The listing builds one solid part. Answer for the finished solid, in the listing's coordinates (mm). Give positions to 0.01 mm unless a question says otherwise; leave off trailing zeros.
```python
from build123d import *

# Parameters (mm, degrees)
SKETCH4_W              = 100
SKETCH4_H              = 50
BODY_DEPTH             = 500
CUT_PROFILE_DEPTH      = 257.173769149
CUT_PROFILE_DEPTH_BACK = 257.173769149
SKETCH6_OUTSIDE_W      = 204.47
SKETCH6_OUTSIDE_H      = 154.47
SKETCH6_OUTSIDE_R      = 4.25
SKETCH6_OUTSIDE_R_2    = 2.5


with BuildPart() as part:
    # Sketch4 → Body (new body)
    with BuildSketch(Plane.XY.offset(250)):
        Rectangle(SKETCH4_W, SKETCH4_H)
    extrude(amount=-BODY_DEPTH)

    # Sketch6 outside → Cut-Profile (cut, two sides: drawn at the far end of the back side and taken through both)
    # profile 1 of 8: a face of its own
    with BuildSketch(Plane.XY.offset(-CUT_PROFILE_DEPTH_BACK)):
        Rectangle(SKETCH6_OUTSIDE_W, SKETCH6_OUTSIDE_H)
        with BuildLine():
            Line((-31.4, -19.7), (-35.8, -19.7))
            ThreePointArc((-35.8, -19.7), (-37.371513222, -18.648341109), (-36.998678382, -16.794524933))
            Line((-36.998678382, -16.794524933), (-31.125524653, -10.954485098))
            ThreePointArc((-31.125524653, -10.954485098), (-29.506885614, -9.877902288), (-27.6, -9.5))
            Line((-27.6, -9.5), (-22.4, -9.5))
            ThreePointArc((-22.4, -9.5), (-20.493114386, -9.877902288), (-18.874475347, -10.954485098))
            Line((-18.874475347, -10.954485098), (-13.001321618, -16.794524933))
            ThreePointArc((-13.001321618, -16.794524933), (-12.628486778, -18.648341109), (-14.2, -19.7))
            Line((-14.2, -19.7), (-18.6, -19.7))
            ThreePointArc((-18.6, -19.7), (-19.589949494, -20.110050506), (-20, -21.1))
            Line((-20, -21.1), (-20, -23.2))
            ThreePointArc((-20, -23.2), (-19.472792206, -24.472792206), (-18.2, -25))
            Line((-18.2, -25), (18.2, -25))
            ThreePointArc((18.2, -25), (19.472792206, -24.472792206), (20, -23.2))
            Line((20, -23.2), (20, -21.1))
            ThreePointArc((20, -21.1), (19.589949494, -20.110050506), (18.6, -19.7))
            Line((18.6, -19.7), (14.2, -19.7))
            ThreePointArc((14.2, -19.7), (12.628486778, -18.648341109), (13.001321618, -16.794524933))
            Line((13.001321618, -16.794524933), (18.874475347, -10.954485098))
            ThreePointArc((18.874475347, -10.954485098), (20.493114386, -9.877902288), (22.4, -9.5))
            Line((22.4, -9.5), (27.6, -9.5))
            ThreePointArc((27.6, -9.5), (29.506885614, -9.877902288), (31.125524653, -10.954485098))
            Line((31.125524653, -10.954485098), (36.998678382, -16.794524933))
            ThreePointArc((36.998678382, -16.794524933), (37.371513222, -18.648341109), (35.8, -19.7))
            Line((35.8, -19.7), (31.4, -19.7))
            ThreePointArc((31.4, -19.7), (30.410050506, -20.110050506), (30, -21.1))
            Line((30, -21.1), (30, -23.2))
            ThreePointArc((30, -23.2), (30.527207794, -24.472792206), (31.8, -25))
            Line((31.8, -25), (45, -25))
            ThreePointArc((45, -25), (48.535533906, -23.535533906), (50, -20))
            Line((50, -20), (50, -6.8))
            ThreePointArc((50, -6.8), (49.472792206, -5.527207794), (48.2, -5))
            Line((48.2, -5), (46.1, -5))
            ThreePointArc((46.1, -5), (45.110050506, -5.410050506), (44.7, -6.4))
            Line((44.7, -6.4), (44.7, -10.8))
            ThreePointArc((44.7, -10.8), (43.648341109, -12.371513222), (41.794524933, -11.998678382))
            Line((41.794524933, -11.998678382), (35.954485098, -6.125524653))
            ThreePointArc((35.954485098, -6.125524653), (34.877902288, -4.506885614), (34.5, -2.6))
            Line((34.5, -2.6), (34.5, 2.6))
            ThreePointArc((34.5, 2.6), (34.877902288, 4.506885614), (35.954485098, 6.125524653))
            Line((35.954485098, 6.125524653), (41.794524933, 11.998678382))
            ThreePointArc((41.794524933, 11.998678382), (43.648341109, 12.371513222), (44.7, 10.8))
            Line((44.7, 10.8), (44.7, 6.4))
            ThreePointArc((44.7, 6.4), (45.110050506, 5.410050506), (46.1, 5))
            Line((46.1, 5), (48.2, 5))
            ThreePointArc((48.2, 5), (49.472792206, 5.527207794), (50, 6.8))
            Line((50, 6.8), (50, 20))
            ThreePointArc((50, 20), (48.535533906, 23.535533906), (45, 25))
            Line((45, 25), (31.8, 25))
            ThreePointArc((31.8, 25), (30.527207794, 24.472792206), (30, 23.2))
            Line((30, 23.2), (30, 21.1))
            ThreePointArc((30, 21.1), (30.410050506, 20.110050506), (31.4, 19.7))
            Line((31.4, 19.7), (35.8, 19.7))
            ThreePointArc((35.8, 19.7), (37.371513222, 18.648341109), (36.998678382, 16.794524933))
            Line((36.998678382, 16.794524933), (31.125524653, 10.954485098))
            ThreePointArc((31.125524653, 10.954485098), (29.506885614, 9.877902288), (27.6, 9.5))
            Line((27.6, 9.5), (22.4, 9.5))
            ThreePointArc((22.4, 9.5), (20.493114386, 9.877902288), (18.874475347, 10.954485098))
            Line((18.874475347, 10.954485098), (13.001321618, 16.794524933))
            ThreePointArc((13.001321618, 16.794524933), (12.628486778, 18.648341109), (14.2, 19.7))
            Line((14.2, 19.7), (18.6, 19.7))
            ThreePointArc((18.6, 19.7), (19.589949494, 20.110050506), (20, 21.1))
            Line((20, 21.1), (20, 23.2))
            ThreePointArc((20, 23.2), (19.472792206, 24.472792206), (18.2, 25))
            Line((18.2, 25), (-18.2, 25))
            ThreePointArc((-18.2, 25), (-19.472792206, 24.472792206), (-20, 23.2))
            Line((-20, 23.2), (-20, 21.1))
            ThreePointArc((-20, 21.1), (-19.589949494, 20.110050506), (-18.6, 19.7))
            Line((-18.6, 19.7), (-14.2, 19.7))
            ThreePointArc((-14.2, 19.7), (-12.628486778, 18.648341109), (-13.001321618, 16.794524933))
            Line((-13.001321618, 16.794524933), (-18.874475347, 10.954485098))
            ThreePointArc((-18.874475347, 10.954485098), (-20.493114386, 9.877902288), (-22.4, 9.5))
            Line((-22.4, 9.5), (-27.6, 9.5))
            ThreePointArc((-27.6, 9.5), (-29.506885614, 9.877902288), (-31.125524653, 10.954485098))
            Line((-31.125524653, 10.954485098), (-36.998678382, 16.794524933))
            ThreePointArc((-36.998678382, 16.794524933), (-37.371513222, 18.648341109), (-35.8, 19.7))
            Line((-35.8, 19.7), (-31.4, 19.7))
            ThreePointArc((-31.4, 19.7), (-30.410050506, 20.110050506), (-30, 21.1))
            Line((-30, 21.1), (-30, 23.2))
            ThreePointArc((-30, 23.2), (-30.527207794, 24.472792206), (-31.8, 25))
            Line((-31.8, 25), (-45, 25))
            ThreePointArc((-45, 25), (-48.535533906, 23.535533906), (-50, 20))
            Line((-50, 20), (-50, 6.8))
            ThreePointArc((-50, 6.8), (-49.472792206, 5.527207794), (-48.2, 5))
            Line((-48.2, 5), (-46.1, 5))
            ThreePointArc((-46.1, 5), (-45.110050506, 5.410050506), (-44.7, 6.4))
            Line((-44.7, 6.4), (-44.7, 10.8))
            ThreePointArc((-44.7, 10.8), (-43.648341109, 12.371513222), (-41.794524933, 11.998678382))
            Line((-41.794524933, 11.998678382), (-35.954485098, 6.125524653))
            ThreePointArc((-35.954485098, 6.125524653), (-34.877902288, 4.506885614), (-34.5, 2.6))
            Line((-34.5, 2.6), (-34.5, -2.6))
            ThreePointArc((-34.5, -2.6), (-34.877902288, -4.506885614), (-35.954485098, -6.125524653))
            Line((-35.954485098, -6.125524653), (-41.794524933, -11.998678382))
            ThreePointArc((-41.794524933, -11.998678382), (-43.648341109, -12.371513222), (-44.7, -10.8))
            Line((-44.7, -10.8), (-44.7, -6.4))
            ThreePointArc((-44.7, -6.4), (-45.110050506, -5.410050506), (-46.1, -5))
            Line((-46.1, -5), (-48.2, -5))
            ThreePointArc((-48.2, -5), (-49.472792206, -5.527207794), (-50, -6.8))
            Line((-50, -6.8), (-50, -20))
            ThreePointArc((-50, -20), (-48.535533906, -23.535533906), (-45, -25))
            Line((-45, -25), (-31.8, -25))
            ThreePointArc((-31.8, -25), (-30.527207794, -24.472792206), (-30, -23.2))
            Line((-30, -23.2), (-30, -21.1))
            ThreePointArc((-30, -21.1), (-30.410050506, -20.110050506), (-31.4, -19.7))
        make_face(mode=Mode.SUBTRACT)
    # profile 2 of 8: a face of its own
    with BuildSketch(Plane.XY.offset(-CUT_PROFILE_DEPTH_BACK)):
        with Locations((25, 0)):
            Circle(SKETCH6_OUTSIDE_R)
    # profile 3 of 8: a face of its own
    with BuildSketch(Plane.XY.offset(-CUT_PROFILE_DEPTH_BACK)):
        with Locations((45, -20)):
            Circle(SKETCH6_OUTSIDE_R_2)
    # profile 4 of 8: a face of its own
    with BuildSketch(Plane.XY.offset(-CUT_PROFILE_DEPTH_BACK)):
        with Locations((45, 20)):
            Circle(SKETCH6_OUTSIDE_R_2)
    # profile 5 of 8: a face of its own
    with BuildSketch(Plane.XY.offset(-CUT_PROFILE_DEPTH_BACK)):
        with Locations((-45, -20)):
            Circle(SKETCH6_OUTSIDE_R_2)
    # profile 6 of 8: a face of its own
    with BuildSketch(Plane.XY.offset(-CUT_PROFILE_DEPTH_BACK)):
        with Locations((-45, 20)):
            Circle(SKETCH6_OUTSIDE_R_2)
    # profile 7 of 8: a face of its own
    with BuildSketch(Plane.XY.offset(-CUT_PROFILE_DEPTH_BACK)):
        with Locations((-25, 0)):
            Circle(SKETCH6_OUTSIDE_R)
    # profile 8 of 8: a face of its own
    with BuildSketch(Plane.XY.offset(-CUT_PROFILE_DEPTH_BACK)):
        with BuildLine():
            Line((14.914213562, 5.685786438), (1.555634919, 19.044365081))
            ThreePointArc((1.555634919, 19.044365081), (0, 19.688730163), (-1.555634919, 19.044365081))
            Line((-1.555634919, 19.044365081), (-14.914213562, 5.685786438))
            ThreePointArc((-14.914213562, 5.685786438), (-15.347759065, 5.03693974), (-15.5, 4.271572875))
            Line((-15.5, 4.271572875), (-15.5, -4.271572875))
            ThreePointArc((-15.5, -4.271572875), (-15.347759065, -5.03693974), (-14.914213562, -5.685786438))
            Line((-14.914213562, -5.685786438), (-1.555634919, -19.044365081))
            ThreePointArc((-1.555634919, -19.044365081), (0, -19.688730163), (1.555634919, -19.044365081))
            Line((1.555634919, -19.044365081), (14.914213562, -5.685786438))
            ThreePointArc((14.914213562, -5.685786438), (15.347759065, -5.03693974), (15.5, -4.271572875))
            Line((15.5, -4.271572875), (15.5, 4.271572875))
            ThreePointArc((15.5, 4.271572875), (15.347759065, 5.03693974), (14.914213562, 5.685786438))
        make_face()
    extrude(amount=CUT_PROFILE_DEPTH + CUT_PROFILE_DEPTH_BACK, mode=Mode.SUBTRACT)


solid = part.part
```
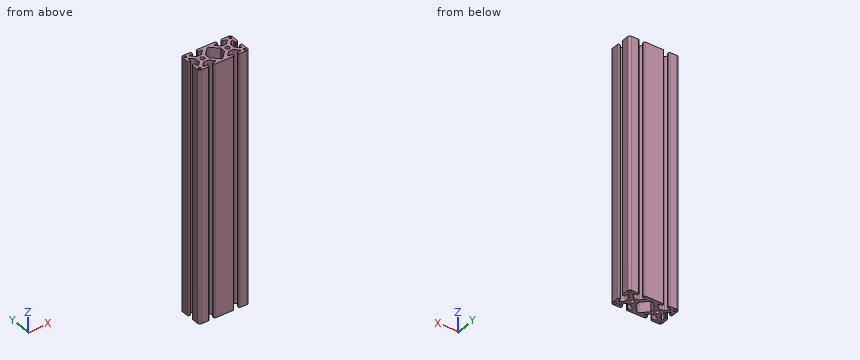
1) Given P1, Ø10, axis at x = -23.5, z = -124.5, coming from the +Y side; P2, Ø5.5, axis at x = 26, z = 82, coming from the +Y side; P3, Ø2.5, axis at y = -21.5, z = -102.5, coming from the -X side; P4, Ø6, axis at x = -23, y = -13.5, coming from the -Z side, each flat-ended and moving along its own axis, determine where each tip first touches the part or whether it passes through.
Geometry says:
P1: stops at y = 24.97
P2: stops at y = 9.63
P3: stops at x = -49.99
P4: passes through
2) Straight lines are drawn through the part: probe 1 along X at (y, z) = (0, -104); probe 2 along Y at (x, z) = (25, 47); probe 3 along X at (y, z) = (-11.5, -131). For each, find the intervals that lie inside material, in ascending order.
Geometry says:
probe 1: x = -34.5 to -29.25, -20.75 to -15.5, 15.5 to 20.75, 29.25 to 34.5
probe 2: y = -9.5 to -4.25, 4.25 to 9.5
probe 3: x = -50 to -44.55, -41.3 to -31.67, -18.33 to -9.1, 9.1 to 18.33, 31.67 to 41.3, 44.55 to 50
3) Find section A-A (z = 77). Count the separate pieces of the cut face and the enclosed holes in it, then the cut area to 3 significant figures.
Geometry says:
separate pieces: 1
enclosed holes: 7
area: 2,510 mm2
